from build123d import *

# Parameters (mm, degrees)
SKETCH004_W             = 85
SKETCH004_H             = 70
SKETCH004_R             = 2.1
PAD003_DEPTH            = 1.6
SKETCH005_W             = 14.05
SKETCH005_H             = 9
PAD004_DEPTH            = 11
SKETCH006_R             = 3.25
SKETCH006_R_2           = 1.05
POCKET001_DEPTH         = 9.5
FILLET_R                = 0.5
POCKET002_DEPTH         = 10
BODY002_PLACEMENT_ANGLE = 90


with BuildPart() as part:
    # Sketch004 → Pad003 (new body)
    with BuildSketch(Plane.XY):
        with Locations((-7.5, 0)):
            Rectangle(SKETCH004_W, SKETCH004_H)
        with Locations((-45, -30)):
            Circle(SKETCH004_R, mode=Mode.SUBTRACT)
        with Locations((30, -30)):
            Circle(SKETCH004_R, mode=Mode.SUBTRACT)
        with Locations((-45, 30)):
            Circle(SKETCH004_R, mode=Mode.SUBTRACT)
        with Locations((30, 30)):
            Circle(SKETCH004_R, mode=Mode.SUBTRACT)
    extrude(amount=PAD003_DEPTH)

    # Sketch005 (on Face10 of Pad003) → Pad004 (join)
    with BuildSketch(Plane.XY.offset(1.6)):
        with Locations((30.975, 15.95)):
            Rectangle(SKETCH005_W, SKETCH005_H)
    extrude(amount=PAD004_DEPTH)

    # Sketch006 (on Face15 of Pad004) → Pocket001 (cut)
    with BuildSketch(Plane.YZ.offset(38)):
        with Locations((15.95, 8.1)):
            Circle(SKETCH006_R)
        with Locations((15.95, 8.1)):
            Circle(SKETCH006_R_2, mode=Mode.SUBTRACT)
    extrude(amount=-POCKET001_DEPTH, mode=Mode.SUBTRACT)

    # Fillet
    fillet_edges = [part.edges().sort_by_distance(p)[0] for p in [
        (38, 14.9, 8.1),
    ]]
    fillet(fillet_edges, radius=FILLET_R)

    # Sketch007 (on Face11 of Fillet) → Pocket002 (cut)
    with BuildSketch(Plane(origin=(23.95, 0, 0), x_dir=(0, -1, 0), z_dir=(-1, 0, 0))):
        with BuildLine():
            ThreePointArc((-11.45, 7.95), (-15.95, 12.45), (-20.45, 7.95))
            Line((-20.45, 7.95), (-20.45, 12.6))
            Line((-20.45, 12.6), (-11.45, 12.6))
            Line((-11.45, 12.6), (-11.45, 7.95))
        make_face()
    extrude(amount=-POCKET002_DEPTH, mode=Mode.SUBTRACT)


with BuildPart() as part_1:
    # Body002 placement: moved
    add(part.part.moved(Location((0, 31, 10.6))).rotate(Axis((0, 31, 10.6), (0, 0, 1)), BODY002_PLACEMENT_ANGLE))


solid = part_1.part
Source: CAD feature listing. Evaluate the final solid. Frame: model axes, mm. A direction names the side the tool comes from. Round coordinates to 2 decimals unless told otherwise and drop trailing zeros. Loops run counter-clockwise (first coordinate to the right, second up) from the corner with the lowest first, then second, coordinate; pieces in that order, holes last. Notation, with made-up numbers: (73.25, 87) -> (90.25, 87) arc R29 ccw to (90.25, 114) -> close; hole circle Ø5 at (29, 76.5). An arc over 180 degrees is marked (long way). Answer as a JSON object with one key per item and string values. Group by question number.
Q1. Contact query for flat-ended pins moving along their axis: P1, Ø4, axis at x = -26.5, z = 14.5, coming from the +Y side; P2, Ø4.5, axis at x = -15, z = 16.5, coming from the -Y side; P3, Ø21, axis at x = -2, y = 40, coming from the +Z side; P4, Ø1.3, axis at x = -9, z = 11, coming from the +Y side. Output: stop coordinate, or through.
Q2. Access query for faces 5 (the flat face through (-16, 67, 12.2)), 6 (the flat face through (-16, 54.95, 18)), 7 (the cylindrical face through (-15.85, 59.88, 23.05)). Directions: +Z, -Z, +X, -X, +Y, -Y. A direction counts if a zero-diameter tool reaches every point of the face in a straight line with its end or side. Return the directions, or none.
Q3. Ray query, line 1 (X direction, y = -14, z = 11); line 2 (Z direction, x = -15, y = 61); line 3 (Z direction, x = 11, y = -14). Return the intervals inside material, ascending. Write a range as from..to.
Q4. Mould query, pull axis X, two halves, no side actions, for faces 1 (the cylindrical face through (31.278, -15.666, 11.389)), 2 (the flat face through (-14.6, 64.95, 23)), 3 (the flat face through (-20.45, 63, 16)), 4 (the flat face through (-16, 59.5, 17)). Classes: pulls with the +X half, pulls with the -X half, needs draft (parallel to the pull), parting line crosses it, or undercut.
Q5. Section query A-A (y = -14). Output: boundary loops of the cut face in (x, z), plus the area to 3 significant figures.
Q6. Section query B-B (x = -30). Output: boundary loops of the cut face in (y, z).
Q7. Section query C-C (y = 57). Output: boundary loops of the cut face in (x, z).
Q8. Section query D-D (x = 21.5). Output: boundary loops of the cut face in (y, z).
Completed:
{
 "1": {"P1": "through", "P2": "y = 54.95", "P3": "z = 12.2", "P4": "y = 66"},
 "2": {"face 5": "-Z, +X, -X, +Y", "face 6": "+Z, +X, -X, -Y", "face 7": "+Z, -Y"},
 "3": {"line 1": "-35..-32.1, -27.9..27.9, 32.1..35", "line 2": "10.6..15.59, 18.25..19.15, 21.81..22.95", "line 3": "10.6..12.2"},
 "4": {"face 1": "undercut", "face 2": "needs draft", "face 3": "pulls with the -X half", "face 4": "undercut"},
 "5": {"outline": "(-35, 10.6) -> (-32.1, 10.6) -> (-32.1, 12.2) -> (-35, 12.2) -> close; (-27.9, 10.6) -> (27.9, 10.6) -> (27.9, 12.2) -> (-27.9, 12.2) -> close; (32.1, 10.6) -> (35, 10.6) -> (35, 12.2) -> (32.1, 12.2) -> close", "area": "98.6 mm²"},
 "6": {"outline": "(-19, 10.6) -> (-16.1, 10.6) -> (-16.1, 12.2) -> (-19, 12.2) -> close; (-11.9, 10.6) -> (58.9, 10.6) -> (58.9, 12.2) -> (-11.9, 12.2) -> close; (63.1, 10.6) -> (66, 10.6) -> (66, 12.2) -> (63.1, 12.2) -> close"},
 "7": {"outline": "(-35, 10.6) -> (35, 10.6) -> (35, 12.2) -> (-11.45, 12.2) -> (-11.45, 18.55) arc R4.5 ccw to (-20.45, 18.55) -> (-20.45, 12.2) -> (-35, 12.2) -> close"},
 "8": {"outline": "(-19, 10.6) -> (66, 10.6) -> (66, 12.2) -> (-19, 12.2) -> close"}
}
